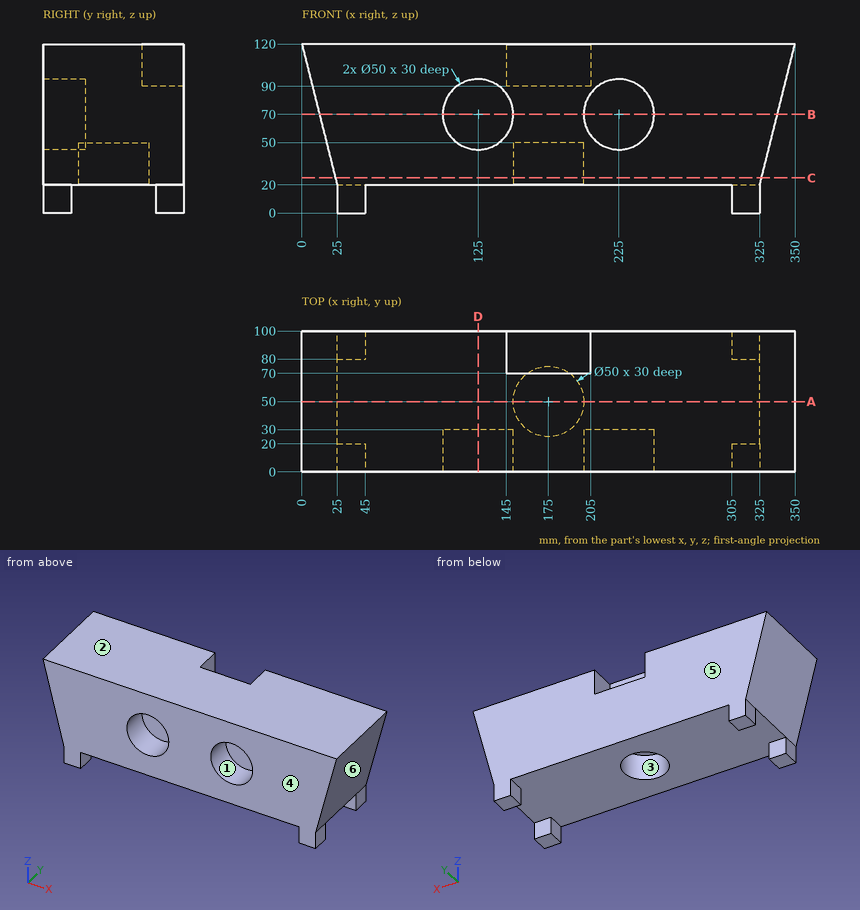
Can you work these out from the drawing? Everything is in mm from the part's minimum corner. A direction names the side the tool comes from. Coordinates: 2 decimals unless noted, no trailing zeros. Loops run counter-clockwise (first coordinate to the right, second up) from the corner with the lowest first, then second, coordinate; pieces in that order, holes last. Notation, with made-up numbers: (26.5, -24.75) - (58.5, -24.75) arc R3 cw to (58.5, -19.75) - close; hole circle Ø6 at (81, -6). An arc over 180 degrees is marked (long way). Put each result on its own line as item: value. Start each with the question number.
Item 1: Suppose I cut it at A-A (y = 50). Please give me the cut outline in (x, z), and give its area (3 significant figures).
Item 2: If I drill on line 1 along Z through (x, y) = (125, 18.25); line 2 along X through (y, z) = (10, 57); line 3 along Y through (x, z) = (175, 32.25), over which ranges is the centre line in solid material (lowest first)?
Item 3: For pin 1 (22 mm diameter, centred on y = 13.5, z = 6, fed in from +X); pin 2 (8 mm diameter, centred on y = 14, z = 57.5, fed in from +X) (3 decimals); pin 3 (8 mm diameter, centred on y = 79, z = 60, fed in from +X), each with a flat end and sliding along its axis, tell me the tip position at first contact or that it passes through.
Item 4: Suppose I cut it at D-D (x = 125). Please give me the cut outline in (y, z), and give its area (3 significant figures).
Item 5: Suppose I cut it at B-B (z = 70). Please give me the cut outline in (x, y).
Item 6: If we mould it in two halves opening along Y, with no side actions, what happens to the marked faces 3, 4, 5 and 6? For each: +Y half, -Y half, draft (parallel to the pull), parting line (faces both ways), or undercut.
Item 7: Which directions (+Z, -Z, +X, -X, +Y, -Y) give clear straight access to the entire face, cutting with the end or side of a thin tool? Please do the marked faces 1 and 2.
Item 8: Suppose I cut it at C-C (z = 25). Please give me the cut outline in (x, y).
Here are the results:
1. outline: (0, 120) - (25, 20) - (150, 20) - (150, 50) - (200, 50) - (200, 20) - (325, 20) - (350, 120) - close
1. area: 31,000 mm²
2. line 1: 20 to 45, 95 to 120
2. line 2: 15.75 to 103.65, 146.35 to 203.65, 246.35 to 334.25
2. line 3: 0 to 25, 75 to 100
3. pin 1: x = 325
3. pin 2: x = 335.375
3. pin 3: x = 336
4. outline: (0, 20) - (100, 20) - (100, 120) - (0, 120) - (0, 95) - (30, 95) - (30, 45) - (0, 45) - close
4. area: 8,500 mm²
5. outline: (12.5, 0) - (100, 0) - (100, 30) - (150, 30) - (150, 0) - (200, 0) - (200, 30) - (250, 30) - (250, 0) - (337.5, 0) - (337.5, 100) - (12.5, 100) - close
6. face 3: undercut
6. face 4: -Y half
6. face 5: +Y half
6. face 6: draft
7. face 1: -Y
7. face 2: +Z, +X, -X, +Y, -Y
8. outline: (23.75, 0) - (326.25, 0) - (326.25, 100) - (23.75, 100) - close; hole circle Ø50 at (175, 50)
